Source: CAD feature listing. Evaluate the final solid. Frame: model axes, mm. A direction names the side the tool comes from. Coordinates: 2 decimals unless noted, no trailing zeros. Order: outer loops, then holes, each group sorted by start corner. A loop starts at its lowest first (then second) coordinate and runs counter-clockwise, first axis right, second up.
```python
from build123d import *

# Parameters (mm, degrees)
SKETCH1_R           = 17
SKETCH1_R_2         = 15
BOSS_EXTRUDE1_DEPTH = 140
SKETCH2_R           = 17
BOSS_EXTRUDE2_DEPTH = 5
SKETCH3_R           = 1.25
CUT_EXTRUDE1_DEPTH  = 18


with BuildPart() as part:
    # Sketch1 → Boss-Extrude1 (new body)
    with BuildSketch(Plane(origin=(0, 0, 0), x_dir=(1, 0, 0), z_dir=(0, 1, 0))):
        Circle(SKETCH1_R)
        Circle(SKETCH1_R_2, mode=Mode.SUBTRACT)
    extrude(amount=BOSS_EXTRUDE1_DEPTH)

    # Sketch2 → Boss-Extrude2 (add)
    with BuildSketch(Plane.XZ):
        Circle(SKETCH2_R)
    extrude(amount=BOSS_EXTRUDE2_DEPTH)

    # Sketch3 → Cut-Extrude1 (cut, through all)
    with BuildSketch(Plane(origin=(0, 0, 0), x_dir=(0, 0, -1), z_dir=(1, 0, 0))):
        with Locations((0, 5.068906343)):
            Circle(SKETCH3_R)
        with Locations((0, 10.668906343)):
            Circle(SKETCH3_R)
        with Locations((-10.429605655, 10.668906343)):
            Circle(SKETCH3_R)
    extrude(amount=CUT_EXTRUDE1_DEPTH, mode=Mode.SUBTRACT)


solid = part.part
```
1. Section query C-C on x = 2. Return loops of the section in (y, z), plus the area to 3 significant figures.
Findings:
outline: (-5, -16.88) - (140, -16.88) - (140, -14.87) - (0, -14.87) - (0, 14.87) - (140, 14.87) - (140, 16.88) - (-5, 16.88) - close
area: 733 mm2
2. Section query B-B on y = 19. Return loops of the section in (x, z), plus the area to 3 significant figures.
Findings:
outline: circle Ø34 at (0, 0); hole circle Ø30 at (0, 0)
area: 201 mm2
3. Ray query, line 1 (Y direction, x = 15.5, z = 0); line 2 (Z direction, x = -0.5, y = 81); line 3 (Y direction, x = 1.5, z = -5). Return the intervals inside material, ascending.
Findings:
line 1: y = -5 to 3.82, 6.32 to 9.42, 11.92 to 140
line 2: z = -16.99 to -14.99, 14.99 to 16.99
line 3: y = -5 to 0
4. Section query A-A on z = 0. Return loops of the section in (x, y).
Findings:
outline: (-17, -5) - (17, -5) - (17, 3.82) - (15, 3.82) - (15, 0) - (-15, 0) - (-15, 140) - (-17, 140) - close; (15, 6.32) - (17, 6.32) - (17, 9.42) - (15, 9.42) - close; (15, 11.92) - (17, 11.92) - (17, 140) - (15, 140) - close
5. Draft query along Y for faces 4 (the face through (6, 140, 14)), 5 (the face through (0, -5, 0)), 6 (the face through (11.83, 10.72, 11.68)). Return one class per face: released by +Y, released by -Y, zero draft, split by the parting line, or undercut.
Findings:
face 4: released by +Y
face 5: released by -Y
face 6: undercut
6. Section query D-D on z = -7. Return loops of the section in (x, y), plus the area to 3 significant figures.
Findings:
outline: (-15.49, -5) - (15.49, -5) - (15.49, 140) - (13.27, 140) - (13.27, 0) - (-13.27, 0) - (-13.27, 140) - (-15.49, 140) - close
area: 778 mm2
7. Pin query (flat end, axial travel): P1, Ø2, axis at y = 10.67, z = 10.43, coming from the -X side; P2, Ø1, axis at x = -12.5, y = 17, coming from the -Z side; P3, Ø4, axis at x = 8, y = 119, coming from the +Z side. Return the tip coordinate at first contact, or that it passes through.
Findings:
P1: stops at x = -14.14
P2: stops at z = -12.04
P3: stops at z = 15.91
8. Access query for faces 1 (the face through (9.139, 68.515, 14.334)), 2 (the face through (0, 0, 0)), 3 (the face through (15.96, 6.31, 0.16)). Directions: +Z, -Z, +X, -X, +Y, -Y. A direction counts if a zero-diameter tool reaches every point of the face in a straight line with its end or side. Return the directions, or none.
Findings:
face 1: +Y, -Y
face 2: +Y
face 3: +X
